Build history of the part. All positions in model axes, mm. Round coordinates to 2 decimals unless told otherwise and drop trailing zeros. Write each loop counter-clockwise with the first axis right and the second up, starting at its lowest first coordinate (ties: lowest second). Pieces come first, ordered by that corner, then holes. Notation, with made-up numbers: M 67,7.25 L 72,7.25 A17 cw 72,25.25 Z; hole C 82.25,30.5 d7. An arc over 180 degrees is marked long. Use a Markdown table: item, result.
from build123d import *

# Parameters (mm, degrees)
SKETCH2_W               = 110
SKETCH2_H               = 110
SKETCH2_W_2             = 100
SKETCH2_H_2             = 100
BOSS_EXTRUDE1_DEPTH     = 89
SKETCH3_W               = 110
SKETCH3_H               = 110
BOSS_EXTRUDE2_DEPTH     = 8
CUT_EXTRUDE1_REACH      = 112
SKETCH6_W               = 60
SKETCH6_H               = 58
SKETCH9_W               = 110
SKETCH9_H               = 110
BOSS_EXTRUDE3_DEPTH     = 3
CUT_EXTRUDE2_REACH      = 63
SKETCH10_R              = 10
BOSS_EXTRUDE4_DEPTH     = 1.5
BOSS_EXTRUDE5_DEPTH     = 1.5
SKETCH14_R              = 3
CUT_EXTRUDE3_DEPTH      = 73
SKETCH15_W              = 2
SKETCH15_H              = 2
CUT_EXTRUDE4_DEPTH      = 113
CUT_EXTRUDE4_DEPTH_BACK = 13
CUT_EXTRUDE5_REACH      = 63
SKETCH16_R              = 2.5
SKETCH17_R              = 14
SKETCH17_R_2            = 11
BOSS_EXTRUDE6_DEPTH     = 7
CUT_EXTRUDE8_REACH      = 7
SKETCH20_R              = 2
SKETCH18_R              = 2
CUT_EXTRUDE6_DEPTH      = 73.5
CUT_EXTRUDE7_REACH      = 63
SKETCH19_R              = 2
SKETCH21_R              = 24
SKETCH21_R_2            = 21
BOSS_EXTRUDE7_DEPTH     = 5
SKETCH23_W              = 110
SKETCH23_H              = 110
CUT_EXTRUDE9_DEPTH      = 58
SKETCH24_W              = 110
SKETCH24_H              = 110
CUT_EXTRUDE10_DEPTH     = 34
CUT_EXTRUDE11_REACH     = 12
SKETCH25_W              = 110
SKETCH25_H              = 110
SKETCH25_W_2            = 100
SKETCH25_H_2            = 100
SKETCH26_R              = 14
CUT_EXTRUDE13_DEPTH     = 7


with BuildPart() as part:
    # Sketch2 → Boss-Extrude1 (new body)
    with BuildSketch(Plane(origin=(0, 0, 0), x_dir=(1, 0, 0), z_dir=(0, 1, 0))):
        Rectangle(SKETCH2_W, SKETCH2_H)
        Rectangle(SKETCH2_W_2, SKETCH2_H_2, mode=Mode.SUBTRACT)
    extrude(amount=BOSS_EXTRUDE1_DEPTH)

    # Sketch3 → Boss-Extrude2 (add)
    with BuildSketch(Plane(origin=(0, 89, 0), x_dir=(1, 0, 0), z_dir=(0, 1, 0))):
        Rectangle(SKETCH3_W, SKETCH3_H)
    extrude(amount=BOSS_EXTRUDE2_DEPTH)

    # Sketch6 → Cut-Extrude1 (cut, up to next)
    with BuildSketch(Plane.XY.offset(55), mode=Mode.PRIVATE) as cut_extrude1_sk1:
        with Locations((0, 29)):
            Rectangle(SKETCH6_W, SKETCH6_H)
    cut_extrude1_tool1 = extrude(cut_extrude1_sk1.sketch, amount=-CUT_EXTRUDE1_REACH, mode=Mode.PRIVATE) & part.part
    add(cut_extrude1_tool1.solids().sort_by_distance((0, 29, 55))[0], mode=Mode.SUBTRACT)

    # Sketch8 → Cut-Revolve1 (revolve, cut)
    with BuildSketch(Plane.XY):
        Polygon((0, 97), (-21, 97), (-21, 94.5), (-16.2, 94.5), (-16.2, 88.5), (0, 88.5), align=None)
    revolve(axis=Axis((0, 0, 0), (0, 1, 0)), mode=Mode.SUBTRACT)

    # Sketch9 → Boss-Extrude3 (add)
    with BuildSketch(Plane.XZ.offset(-58)):
        Rectangle(SKETCH9_W, SKETCH9_H)
    extrude(amount=-BOSS_EXTRUDE3_DEPTH)

    # Sketch10 → Cut-Extrude2 (cut, up to next)
    with BuildSketch(Plane(origin=(0, 61, 0), x_dir=(1, 0, 0), z_dir=(0, 1, 0)), mode=Mode.PRIVATE) as cut_extrude2_sk1:
        Circle(SKETCH10_R)
    cut_extrude2_tool1 = extrude(cut_extrude2_sk1.sketch, amount=-CUT_EXTRUDE2_REACH, mode=Mode.PRIVATE) & part.part
    add(cut_extrude2_tool1.solids().sort_by_distance((0, 61, 0))[0], mode=Mode.SUBTRACT)

    # Sketch11 → Boss-Extrude4 (add, symmetric)
    with BuildSketch(Plane.XY):
        Polygon((-50, 89), (-35, 89), (-50, 69), align=None)
    boss_extrude4 = extrude(amount=BOSS_EXTRUDE4_DEPTH, both=True)

    # Mirror1: Boss-Extrude4 across plane
    add(boss_extrude4.mirror(Plane(origin=(0, 0, 0), x_dir=(0, 0, 1), z_dir=(1, 0, 0))))

    # Sketch12 → Boss-Extrude5 (add, symmetric)
    with BuildSketch(Plane(origin=(0, 0, 0), x_dir=(0, 0, -1), z_dir=(1, 0, 0))):
        Polygon((-35, 89), (-50, 89), (-50, 69), align=None)
    boss_extrude5 = extrude(amount=BOSS_EXTRUDE5_DEPTH, both=True)

    # Mirror2: Boss-Extrude5 across plane
    add(boss_extrude5.mirror(Plane.XY))

    # Sketch14 → Cut-Extrude3 (cut)
    with BuildSketch(Plane(origin=(0, 97, 0), x_dir=(1, 0, 0), z_dir=(0, 1, 0))):
        with Locations((40, 40)):
            Circle(SKETCH14_R)
        with Locations((-40, -40)):
            Circle(SKETCH14_R)
    extrude(amount=-CUT_EXTRUDE3_DEPTH, mode=Mode.SUBTRACT)

    # Sketch15 → Cut-Extrude4 (cut, two sides)
    with BuildSketch(Plane(origin=(-50, 0, 0), x_dir=(0, 0, -1), z_dir=(1, 0, 0))) as cut_extrude4_sk:
        with Locations((-24, 62)):
            Rectangle(SKETCH15_W, SKETCH15_H)
        with Locations((24, 62)):
            Rectangle(SKETCH15_W, SKETCH15_H)
    extrude(amount=CUT_EXTRUDE4_DEPTH, mode=Mode.SUBTRACT)
    extrude(cut_extrude4_sk.sketch, amount=-CUT_EXTRUDE4_DEPTH_BACK, mode=Mode.SUBTRACT)

    # Sketch16 → Cut-Extrude5 (cut, up to next)
    with BuildSketch(Plane(origin=(0, 61, 0), x_dir=(1, 0, 0), z_dir=(0, 1, 0)), mode=Mode.PRIVATE) as cut_extrude5_sk1:
        with Locations((-14, 11.15)):
            Circle(SKETCH16_R)
    cut_extrude5_tool1 = extrude(cut_extrude5_sk1.sketch, amount=-CUT_EXTRUDE5_REACH, mode=Mode.PRIVATE) & part.part
    add(cut_extrude5_tool1.solids().sort_by_distance((-14, 61, -11.15))[0], mode=Mode.SUBTRACT)
    # Sketch16 → Cut-Extrude5 (cut, up to next)
    with BuildSketch(Plane(origin=(0, 61, 0), x_dir=(1, 0, 0), z_dir=(0, 1, 0)), mode=Mode.PRIVATE) as cut_extrude5_sk2:
        with Locations((-14, -28.85)):
            Circle(SKETCH16_R)
    cut_extrude5_tool2 = extrude(cut_extrude5_sk2.sketch, amount=-CUT_EXTRUDE5_REACH, mode=Mode.PRIVATE) & part.part
    add(cut_extrude5_tool2.solids().sort_by_distance((-14, 61, 28.85))[0], mode=Mode.SUBTRACT)
    # Sketch16 → Cut-Extrude5 (cut, up to next)
    with BuildSketch(Plane(origin=(0, 61, 0), x_dir=(1, 0, 0), z_dir=(0, 1, 0)), mode=Mode.PRIVATE) as cut_extrude5_sk3:
        with Locations((14, -28.85)):
            Circle(SKETCH16_R)
    cut_extrude5_tool3 = extrude(cut_extrude5_sk3.sketch, amount=-CUT_EXTRUDE5_REACH, mode=Mode.PRIVATE) & part.part
    add(cut_extrude5_tool3.solids().sort_by_distance((14, 61, 28.85))[0], mode=Mode.SUBTRACT)
    # Sketch16 → Cut-Extrude5 (cut, up to next)
    with BuildSketch(Plane(origin=(0, 61, 0), x_dir=(1, 0, 0), z_dir=(0, 1, 0)), mode=Mode.PRIVATE) as cut_extrude5_sk4:
        with Locations((14, 11.15)):
            Circle(SKETCH16_R)
    cut_extrude5_tool4 = extrude(cut_extrude5_sk4.sketch, amount=-CUT_EXTRUDE5_REACH, mode=Mode.PRIVATE) & part.part
    add(cut_extrude5_tool4.solids().sort_by_distance((14, 61, -11.15))[0], mode=Mode.SUBTRACT)

    # Sketch17 → Boss-Extrude6 (add)
    with BuildSketch(Plane(origin=(0, 61, 0), x_dir=(1, 0, 0), z_dir=(0, 1, 0))):
        Circle(SKETCH17_R)
        Circle(SKETCH17_R_2, mode=Mode.SUBTRACT)
    extrude(amount=BOSS_EXTRUDE6_DEPTH)

    # Sketch20 → Cut-Extrude8 (cut, up to next)
    with BuildSketch(Plane.XY.offset(-50), mode=Mode.PRIVATE) as cut_extrude8_sk1:
        with Locations((10, 48)):
            Circle(SKETCH20_R)
    cut_extrude8_tool1 = extrude(cut_extrude8_sk1.sketch, amount=-CUT_EXTRUDE8_REACH, mode=Mode.PRIVATE) & part.part
    add(cut_extrude8_tool1.solids().sort_by_distance((10, 48, -50))[0], mode=Mode.SUBTRACT)
    # Sketch20 → Cut-Extrude8 (cut, up to next)
    with BuildSketch(Plane.XY.offset(-50), mode=Mode.PRIVATE) as cut_extrude8_sk2:
        with Locations((-10, 48)):
            Circle(SKETCH20_R)
    cut_extrude8_tool2 = extrude(cut_extrude8_sk2.sketch, amount=-CUT_EXTRUDE8_REACH, mode=Mode.PRIVATE) & part.part
    add(cut_extrude8_tool2.solids().sort_by_distance((-10, 48, -50))[0], mode=Mode.SUBTRACT)

    # Sketch18 → Cut-Extrude6 (cut, symmetric)
    with BuildSketch(Plane(origin=(0, 0, 0), x_dir=(0, 0, -1), z_dir=(1, 0, 0))):
        with Locations((10, 48)):
            Circle(SKETCH18_R)
        with Locations((-10, 48)):
            Circle(SKETCH18_R)
    extrude(amount=CUT_EXTRUDE6_DEPTH, both=True, mode=Mode.SUBTRACT)

    # Sketch19 → Cut-Extrude7 (cut, up to next)
    with BuildSketch(Plane(origin=(0, 61, 0), x_dir=(1, 0, 0), z_dir=(0, 1, 0)), mode=Mode.PRIVATE) as cut_extrude7_sk1:
        with Locations((40, 10)):
            Circle(SKETCH19_R)
    cut_extrude7_tool1 = extrude(cut_extrude7_sk1.sketch, amount=-CUT_EXTRUDE7_REACH, mode=Mode.PRIVATE) & part.part
    add(cut_extrude7_tool1.solids().sort_by_distance((40, 61, -10))[0], mode=Mode.SUBTRACT)
    # Sketch19 → Cut-Extrude7 (cut, up to next)
    with BuildSketch(Plane(origin=(0, 61, 0), x_dir=(1, 0, 0), z_dir=(0, 1, 0)), mode=Mode.PRIVATE) as cut_extrude7_sk2:
        with Locations((40, -10)):
            Circle(SKETCH19_R)
    cut_extrude7_tool2 = extrude(cut_extrude7_sk2.sketch, amount=-CUT_EXTRUDE7_REACH, mode=Mode.PRIVATE) & part.part
    add(cut_extrude7_tool2.solids().sort_by_distance((40, 61, 10))[0], mode=Mode.SUBTRACT)
    # Sketch19 → Cut-Extrude7 (cut, up to next)
    with BuildSketch(Plane(origin=(0, 61, 0), x_dir=(1, 0, 0), z_dir=(0, 1, 0)), mode=Mode.PRIVATE) as cut_extrude7_sk3:
        with Locations((-40, -10)):
            Circle(SKETCH19_R)
    cut_extrude7_tool3 = extrude(cut_extrude7_sk3.sketch, amount=-CUT_EXTRUDE7_REACH, mode=Mode.PRIVATE) & part.part
    add(cut_extrude7_tool3.solids().sort_by_distance((-40, 61, 10))[0], mode=Mode.SUBTRACT)
    # Sketch19 → Cut-Extrude7 (cut, up to next)
    with BuildSketch(Plane(origin=(0, 61, 0), x_dir=(1, 0, 0), z_dir=(0, 1, 0)), mode=Mode.PRIVATE) as cut_extrude7_sk4:
        with Locations((-40, 10)):
            Circle(SKETCH19_R)
    cut_extrude7_tool4 = extrude(cut_extrude7_sk4.sketch, amount=-CUT_EXTRUDE7_REACH, mode=Mode.PRIVATE) & part.part
    add(cut_extrude7_tool4.solids().sort_by_distance((-40, 61, -10))[0], mode=Mode.SUBTRACT)
    # Sketch19 → Cut-Extrude7 (cut, up to next)
    with BuildSketch(Plane(origin=(0, 61, 0), x_dir=(1, 0, 0), z_dir=(0, 1, 0)), mode=Mode.PRIVATE) as cut_extrude7_sk5:
        with Locations((10, 40)):
            Circle(SKETCH19_R)
    cut_extrude7_tool5 = extrude(cut_extrude7_sk5.sketch, amount=-CUT_EXTRUDE7_REACH, mode=Mode.PRIVATE) & part.part
    add(cut_extrude7_tool5.solids().sort_by_distance((10, 61, -40))[0], mode=Mode.SUBTRACT)
    # Sketch19 → Cut-Extrude7 (cut, up to next)
    with BuildSketch(Plane(origin=(0, 61, 0), x_dir=(1, 0, 0), z_dir=(0, 1, 0)), mode=Mode.PRIVATE) as cut_extrude7_sk6:
        with Locations((-10, 40)):
            Circle(SKETCH19_R)
    cut_extrude7_tool6 = extrude(cut_extrude7_sk6.sketch, amount=-CUT_EXTRUDE7_REACH, mode=Mode.PRIVATE) & part.part
    add(cut_extrude7_tool6.solids().sort_by_distance((-10, 61, -40))[0], mode=Mode.SUBTRACT)

    # Sketch21 → Boss-Extrude7 (add)
    with BuildSketch(Plane(origin=(0, 97, 0), x_dir=(1, 0, 0), z_dir=(0, 1, 0))):
        Circle(SKETCH21_R)
        Circle(SKETCH21_R_2, mode=Mode.SUBTRACT)
    extrude(amount=BOSS_EXTRUDE7_DEPTH)

    # Sketch23 → Cut-Extrude9 (cut)
    with BuildSketch(Plane.XZ):
        Rectangle(SKETCH23_W, SKETCH23_H)
    extrude(amount=-CUT_EXTRUDE9_DEPTH, mode=Mode.SUBTRACT)

    # Sketch24 → Cut-Extrude10 (cut)
    with BuildSketch(Plane(origin=(0, 102, 0), x_dir=(1, 0, 0), z_dir=(0, 1, 0))):
        Rectangle(SKETCH24_W, SKETCH24_H)
    extrude(amount=-CUT_EXTRUDE10_DEPTH, mode=Mode.SUBTRACT)

    # Sketch25 → Cut-Extrude11 (cut, up to next)
    with BuildSketch(Plane(origin=(0, 68, 0), x_dir=(1, 0, 0), z_dir=(0, 1, 0)), mode=Mode.PRIVATE) as cut_extrude11_sk1:
        Rectangle(SKETCH25_W, SKETCH25_H)
        Rectangle(SKETCH25_W_2, SKETCH25_H_2, mode=Mode.SUBTRACT)
    cut_extrude11_tool1 = extrude(cut_extrude11_sk1.sketch, amount=-CUT_EXTRUDE11_REACH, mode=Mode.PRIVATE) & part.part
    add(cut_extrude11_tool1.solids().sort_by_distance((0, 68, 53.444365))[0], mode=Mode.SUBTRACT)

    # Sketch26 → Cut-Extrude13 (cut)
    with BuildSketch(Plane(origin=(0, 68, 0), x_dir=(1, 0, 0), z_dir=(0, 1, 0))):
        Circle(SKETCH26_R)
    extrude(amount=-CUT_EXTRUDE13_DEPTH, mode=Mode.SUBTRACT)


solid = part.part
Q1. Cut at D-D on x = -40. Give the cut face in (y, z).
Response values:
| item | result |
|---|---|
| outline | M 58,-50 L 61,-50 L 61,-12 L 58,-12 Z; M 58,-8 L 61,-8 L 61,8 L 58,8 Z; M 58,12 L 61,12 L 61,37 L 58,37 Z; M 58,43 L 61,43 L 61,50 L 58,50 Z |
Q2. Two-plate mould, pull along Z, no slides. Class faces 1 (the flat face through (-1, 60, 50)), 2 (the flat face through (1, 61, 12)), 3 (the cylindrical face through (37.79, 59.52, -42.03)): +Z half, -Z half, draft (parallel to the pull), parting line (faces both ways), or undercut.
Response values:
| item | result |
|---|---|
| face 1 | +Z half |
| face 2 | draft |
| face 3 | undercut |
Q3. Drill centre lines: L1, parallel to X at y = 60.2, z = -40; L2, parallel to Z at x = -14, y = 59.9; L3, parallel to X at y = 60.25, z = 28.85. Where is each one in solid material? Low to high.
Response values:
| item | result |
|---|---|
| L1 | x = -50 to -12, -8 to 8, 12 to 37, 43 to 50 |
| L2 | z = -50 to -13.65, -8.65 to 26.35, 31.35 to 50 |
| L3 | x = -50 to -16.5, -11.5 to 11.5, 16.5 to 50 |
Q4. Cut at B-B on z = 28.85. Give the cut face in (x, y).
Response values:
| item | result |
|---|---|
| outline | M -50,58 L -16.5,58 L -16.5,61 L -50,61 Z; M -11.5,58 L 11.5,58 L 11.5,61 L -11.5,61 Z; M 16.5,58 L 50,58 L 50,61 L 16.5,61 Z |
Q5. Cut at C-C on y = 58.6. Count the separate pieces of the cut face and the enclosed holes in it, and give its area (3 significant figures).
Response values:
| item | result |
|---|---|
| separate pieces | 1 |
| enclosed holes | 13 |
| area | 9,480 mm2 |
Q6. Cut at A-A on x = 14. Give the cut face in (y, z), and give its area (3 significant figures).
Response values:
| item | result |
|---|---|
| outline | M 58,-50 L 61,-50 L 61,-13.65 L 58,-13.65 Z; M 58,-8.65 L 61,-8.65 L 61,26.35 L 58,26.35 Z; M 58,31.35 L 61,31.35 L 61,50 L 58,50 Z |
| area | 270 mm2 |
